Autodesk Inventor part; units mm, degrees
ref_plane "YZ Plane" through (0, 0, 0) normal (1, 0, 0) x (0, 1, 0)
ref_plane "XZ Plane" through (0, 0, 0) normal (0, 1, 0) x (-1, 0, 0)
ref_plane "XY Plane" through (0, 0, 0) normal (0, 0, 1) x (1, 0, 0)
sketch "Sketch1" plane through (0, 0, 0) normal (0, 0, 1) x (1, 0, 0)
  arc A0 (45.9619, 45.9619) -> (0, 65) centre (0, 0) ccw construction
  arc A1 (56.5685, 56.5685) -> (0, 80) centre (0, 0) ccw
  arc A2 (35.3553, 35.3553) -> (0, 50) centre (0, 0) ccw
  arc A3 (35.3553, 35.3553) -> (56.5685, 56.5685) centre (45.9619, 45.9619) ccw
  arc A4 (0, 80) -> (0, 50) centre (0, 65) ccw
  line L0 (0, 65) -> (0, 0)
  line L1 (0, 0) -> (45.9619, 45.9619)
  circle A5 centre (0, 65) radius 5
  circle A6 centre (45.9619, 45.9619) radius 5
  dimension "d0" = 45
  dimension "d1" = 50
  dimension "d2" = 80
  dimension "d3" = 10
  dimension "d4" = 10
extrude "Extrusion1" add sketch "Sketch1" along normal blind 7.9375 contours A3 A2 A4 A1
properties part number "Support" material "Steel, Mild"
Input: part model. Units: mm. Frame: model coordinates. Give positions to 0.01 mm unless a question says otherwise; leave off trailing zeros. Order: outer loops, then holes, each group sorted by start corner. A loop starts at its lowest first (then second) coordinate and runs counter-clockwise, first axis right, second up. Notation, with made-up numbers: (65, 20) - (79, 20) arc R10 ccw to (79, 28) - close; hole circle Ø7 at (49.25, 33). An arc over 180 degrees is marked (long way). Put each result on its own line as item: value.
Item 1: Ray query, L1, parallel to Y at x = 0, z = 4.25; L2, parallel to X at y = 65, z = 3.5; L3, parallel to Y at x = -1, z = 4.75. Return the intervals inside material, ascending. Write a range as from..to.
Found:
L1: y = 50..60, 70..80
L2: x = -15..-5, 5..46.64
L3: y = 50.03..60.1, 69.9..79.97
Item 2: Contact query for flat-ended pins moving along their axis: pin 1 (1 mm diameter, centred on x = 31, z = 2.5, fed in from -Y); pin 2 (3 mm diameter, centred on y = 42.5, z = 3.5, fed in from -X); pin 3 (3 mm diameter, centred on y = 74.5, z = 6.5, fed in from +X). Output: stop coordinate, or through.
Found:
pin 1: stops at y = 38.83
pin 2: stops at x = 23.75
pin 3: stops at x = 32.73
Item 3: Section query C-C, the plane x = 17. Return loops of the section in (y, z), then the cut area to 3 significant figures.
Found:
outline: (47.02, 0) - (78.17, 0) - (78.17, 7.94) - (47.02, 7.94) - close
area: 247 mm^2
Item 4: Draft query along X for faces 1 (the cylindrical face through (-0.651, 60.043, 3.913)), 2 (the flat face through (22, 56, 0)), 3 (the cylindrical face through (18.88, 46.3, 3.91)), 4 (the cylindrical face through (48.65, 41.746, 3.913)). Return one class per face: +X half, -X half, draft (parallel to the pull), parting line (faces both ways), or undercut.
Found:
face 1: undercut
face 2: draft
face 3: -X half
face 4: undercut
Item 5: Section query A-A, the plane y = 65. Return loops of the section in (x, z), then the cut area to 3 significant figures.
Found:
outline: (-15, 0) - (-5, 0) - (-5, 7.94) - (-15, 7.94) - close; (5, 0) - (46.64, 0) - (46.64, 7.94) - (5, 7.94) - close
area: 410 mm^2
Item 6: Section query B-B, the plane z = 4.75. Return loops of the section in (x, y), then the cut area to 3 significant figures.
Found:
outline: (0, 50) arc R50 cw to (35.36, 35.36) arc R15 ccw to (56.57, 56.57) arc R80 ccw to (0, 80) arc R15 ccw to start; hole circle Ø10 at (0, 65); hole circle Ø10 at (45.96, 45.96)
area: 2,080 mm^2
Item 7: Section query D-D, the plane y = 49. Return loops of the section in (x, z), then the cut area to 3 significant figures.
Found:
outline: (9.95, 0) - (41.99, 0) - (41.99, 7.94) - (9.95, 7.94) - close; (49.93, 0) - (60.65, 0) - (60.65, 7.94) - (49.93, 7.94) - close
area: 339 mm^2
